```python
from build123d import *

# Parameters (mm, degrees)
F0_W     = 100
F0_H     = 100
F1_DEPTH = 1
F2_R     = 5
F3_R     = 1.676803
F4_DEPTH = 25
F5_R     = 33.189229
F6_DEPTH = 30
F7_R     = 25.904807
F8_DEPTH = 25
F9_R     = 7


with BuildPart() as f1:
    # F0 (on Top) → F1 (new body)
    with BuildSketch(Plane.XY):
        Rectangle(F0_W, F0_H)
    extrude(amount=F1_DEPTH)

    # F2
    f2_edges = [f1.edges().sort_by_distance(p)[0] for p in [
        (50, -50, 0.5),
        (-50, -50, 0.5),
        (-50, 50, 0.5),
        (50, 50, 0.5),
    ]]
    fillet(f2_edges, radius=F2_R)

    # F3 (on face) → F4 (cut)
    with BuildSketch(Plane.XY.offset(1)):
        with Locations((45, 45)):
            Circle(F3_R)
        with Locations((-45, 45)):
            Circle(F3_R)
        with Locations((-45, -45)):
            Circle(F3_R)
        with Locations((45, -45)):
            Circle(F3_R)
    extrude(amount=-F4_DEPTH, mode=Mode.SUBTRACT)

    # F5 (on face) → F6 (join)
    with BuildSketch(Plane.XY.offset(1)):
        Circle(F5_R)
    extrude(amount=F6_DEPTH)

    # F7 (on face) → F8 (cut)
    with BuildSketch(Plane(origin=(0, 0, 0), x_dir=(1, 0, 0), z_dir=(0, 0, -1))):
        Circle(F7_R)
    extrude(amount=-F8_DEPTH, mode=Mode.SUBTRACT)

    # F9
    f9_edges = [f1.edges().sort_by_distance(p)[0] for p in [
        (-33.189229, 0, 31),
        (-25.904807, 0, 25),
    ]]
    fillet(f9_edges, radius=F9_R)


solid = f1.part
```
Input: part model. Units: mm. Frame: model coordinates. A direction names the side the tool comes from. Round coordinates to 2 decimals unless told otherwise and drop trailing zeros. Loops run counter-clockwise (first coordinate to the right, second up) from the corner with the lowest first, then second, coordinate; pieces in that order, holes last. Notation, with made-up numbers: M 68,71.5 L 86,71.5 A23 cw 86,85.5 Z; hole C -33,-38 d9. An arc over 180 degrees is marked long. Answer in a Markdown table with one row per item. Add a question column.
1. Section B-B (z = 16). Output: boundary loops of the cut face in (x, y).
2. Set-up query: faces 4 (the face through (-34, 1, 1)), 5 (the face through (24.71, -7.78, 8.87)), 6 (the face through (-44.099, 46.414, 0.507)). Return all of +Z, -Z, +X, -X, +Y, -Y with unobstructed straight access to the full face (end or side cutting, diameter ignored); none if empty.
3. Mould query, pull axis Y, two halves, no side actions, for faces 1 (the face through (-48.57, 48.5, 0.51)), 2 (the face through (0, 0, 25)), 3 (the face through (17.842, 27.985, 12.339)). Classes: released by +Y, released by -Y, zero draft, split by the parting line, or undercut.
4. Section A-A (x = 0). Output: boundary loops of the cut face in (y, z), and give its area (3 significant figures).
5. Ray query, probe 1 along Y at (x, z) = (45, 0.3); probe 2 along Y at (x, z) = (0, 4.25); probe 3 along Z at (x, y) = (2, -2). Return the intervals inside material, ascending.
6. Section D-D (z = 29). Output: boundary loops of the cut face in (x, y).
7. Section C-C (y = -39). Output: boundary loops of the cut face in (x, z), and give its area (3 significant figures).
8. Contact query for flat-ended pins moving along their axis: pin 1 (4.5 mm diameter, centred on x = 45, y = 45, fed in from +Z); pin 2 (1.5 mm diameter, centred on y = 16, z = 23.5, fed in from +X); pin 3 (1 mm diameter, centred on x = -19.5, y = -22, fed in from +Z). Output: stop coordinate, or through.
Values follow:
| question | item | result |
|---|---|---|
| 1 | outline | C 0,0 d66.38; hole C 0,0 d51.81 |
| 2 | face 4 | +Z |
| 2 | face 5 | -Z |
| 2 | face 6 | +Z, -Z |
| 3 | face 1 | released by +Y |
| 3 | face 2 | undercut |
| 3 | face 3 | split by the parting line |
| 4 | outline | M -50,0 L -25.9,0 L -25.9,18 A7 cw -18.9,25 L 18.9,25 A7 cw 25.9,18 L 25.9,0 L 50,0 L 50,1 L 33.19,1 L 33.19,24 A7 ccw 26.19,31 L -26.19,31 A7 ccw -33.19,24 L -33.19,1 L -50,1 Z |
| 4 | area | 796 mm^2 |
| 5 | probe 1 | -50 to -46.68, -43.32 to 43.32, 46.68 to 50 |
| 5 | probe 2 | -33.19 to -25.9, 25.9 to 33.19 |
| 5 | probe 3 | 25 to 31 |
| 6 | outline | C 0,0 d62.18 |
| 7 | outline | M -50,0 L 50,0 L 50,1 L -50,1 Z |
| 7 | area | 100 mm^2 |
| 8 | pin 1 | z = 1 |
| 8 | pin 2 | x = 29.48 |
| 8 | pin 3 | z = 30.45 |
